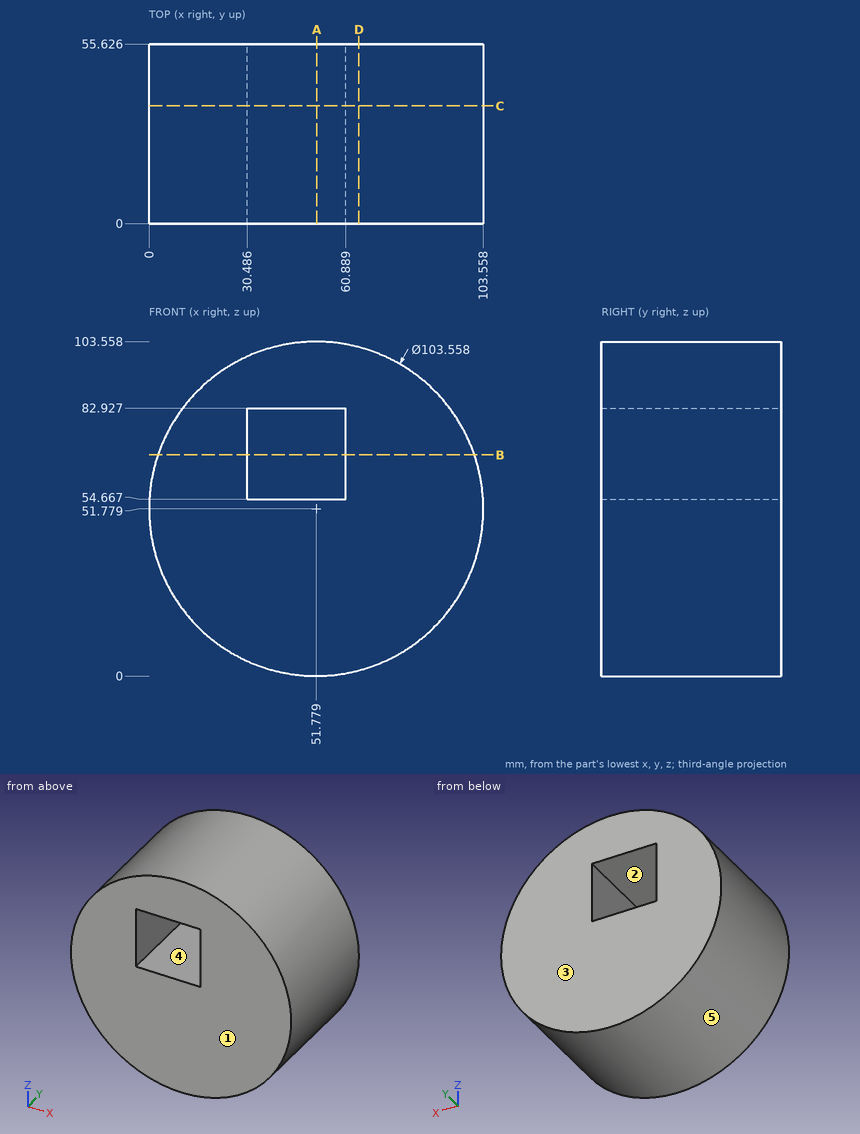
Could you check a few things on this drawing? It's one solid part, dimensions in mm from its lowest x, y, z. A direction names the side the tool comes from. Coordinates: 2 decimals unless noted, no trailing zeros. Loops run counter-clockwise (first coordinate to the right, second up) from the corner with the lowest first, then second, coordinate; pieces in that order, holes last. Notation, with made-up numbers: (-15, -21) - (26, -21) arc R24 ccw to (26, 15) - close; hole circle Ø3 at (3.5, -6.5). An arc over 180 degrees is marked (long way). Return JSON: item names as keys, results as strings. Group by question number.
Item 1: We'd pull the mould along Z, two halves only. Please class the marked faces 3, 4 and 5: +Z half, -Z half, draft (parallel to the pull), parting line (faces both ways), or undercut.
Item 2: If we section it at B-B on z = 68.5: Write out the boundary of the cut face in (x, y) (1 decimal).
Item 3: If we section it at D-D on x = 65: Write out the boundary of the cut face in (y, z).
Item 4: If we section it at C-C on y = 36.5: Write out the boundary of the cut face in (x, z) (1 decimal).
Item 5: On a 3-axis mill with a long thin cutter (end or side, diameter ignored), from which of +Z, -Z, +X, -X, +Y, -Y can I reach the whole of each face in a straight line? I mean the marked faces 1 and 2. Say none if no direction works.
Item 6: Will these pins go through, and if not, where does the flat tip stop? P1, Ø22.5, axis at y = 26, z = 67.5, coming from the -X side; P2, Ø1.5, axis at y = 37.5, z = 24, coming from the +X side; P3, Ø1, axis at y = 9.5, z = 57.5, coming from the -X side.
Item 7: If we section it at A-A on x = 52: Write out the boundary of the cut face in (y, z).
Item 8: I need wall thicknesses on line 1 (Z direction, x = 55.5, y = 36.5); line 2 (Z direction, x = 58, y = 3.5) (1 decimal); line 3 (X direction, y = 50.5, z = 63) (1 decimal). Which ranges of each line are inside material? Lowest first, please. Write a range as from..to.
Calculated:
{
 "1": {"face 3": "draft", "face 4": "undercut", "face 5": "parting line"},
 "2": {"outline": "(2.8, 0) - (30.5, 0) - (30.5, 55.6) - (2.8, 55.6) - close; (60.9, 0) - (100.8, 0) - (100.8, 55.6) - (60.9, 55.6) - close"},
 "3": {"outline": "(0, 1.72) - (55.63, 1.72) - (55.63, 101.84) - (0, 101.84) - close"},
 "4": {"outline": "circle Ø103.6 at (51.8, 51.8); hole (30.5, 54.7) - (60.9, 54.7) - (60.9, 82.9) - (30.5, 82.9) - close"},
 "5": {"face 1": "+Z, -Z, +X, -X, -Y", "face 2": "+Y, -Y"},
 "6": {"P1": "stops at x = 0.19", "P2": "stops at x = 95.94", "P3": "stops at x = 0.26"},
 "7": {"outline": "(0, 0) - (55.63, 0) - (55.63, 54.67) - (0, 54.67) - close; (0, 82.93) - (55.63, 82.93) - (55.63, 103.56) - (0, 103.56) - close"},
 "8": {"line 1": "z = 0.13..54.67, 82.93..103.42", "line 2": "z = 0.4..54.7, 82.9..103.2", "line 3": "x = 1.2..30.5, 60.9..102.3"}
}
